```python
from build123d import *

# Parameters (mm, degrees)
BOSS_EXTRUDE1_DEPTH  = 25
CUT_EXTRUDE1_DEPTH   = 23
BOSS_EXTRUDE2_DEPTH  = 30
RIB5_REACH           = 157.804
SKETCH9_WALL_W       = 390.44961144
SKETCH9_WALL_H       = 50
FILLET2_R            = 2
FILLET3_R            = 2
FILLET2_OF_MIRROR1_R = 2
FILLET3_OF_MIRROR1_R = 2
RIB6_REACH           = 157.804
SKETCH10_WALL_W      = 362.214279798
SKETCH10_WALL_H      = 90
FILLET4_R            = 2
FILLET4_OF_MIRROR3_R = 2
SKETCH11_W           = 95
SKETCH11_H           = 63
CUT_EXTRUDE2_DEPTH   = 30
CUT_EXTRUDE3_DEPTH   = 1
SKETCH14_R           = 9
CUT_EXTRUDE4_DEPTH   = 5
FILLET6_R            = 3
FILLET7_R            = 3
CUT_EXTRUDE5_REACH   = 157.804
SKETCH21_R           = 3


with BuildPart() as part:
    # Sketch1 → Boss-Extrude1 (new body)
    with BuildSketch(Plane.XY):
        with BuildLine():
            Line((-119, 35), (-58.5, 35))
            ThreePointArc((-58.5, 35), (-54.257359313, 36.757359313), (-52.5, 41))
            Line((-52.5, 41), (-52.5, 69))
            ThreePointArc((-52.5, 69), (-50.742640687, 73.242640687), (-46.5, 75))
            Line((-46.5, 75), (46.5, 75))
            ThreePointArc((46.5, 75), (50.742640687, 73.242640687), (52.5, 69))
            Line((52.5, 69), (52.5, 41))
            ThreePointArc((52.5, 41), (54.257359313, 36.757359313), (58.5, 35))
            Line((58.5, 35), (119, 35))
            ThreePointArc((119, 35), (123.242640687, 33.242640687), (125, 29))
            Line((125, 29), (125, -29))
            ThreePointArc((125, -29), (123.242640687, -33.242640687), (119, -35))
            Line((119, -35), (58.5, -35))
            ThreePointArc((58.5, -35), (54.257359313, -36.757359313), (52.5, -41))
            Line((52.5, -41), (52.5, -69))
            ThreePointArc((52.5, -69), (50.742640687, -73.242640687), (46.5, -75))
            Line((46.5, -75), (-46.5, -75))
            ThreePointArc((-46.5, -75), (-50.742640687, -73.242640687), (-52.5, -69))
            Line((-52.5, -69), (-52.5, -41))
            ThreePointArc((-52.5, -41), (-54.257359313, -36.757359313), (-58.5, -35))
            Line((-58.5, -35), (-119, -35))
            ThreePointArc((-119, -35), (-123.242640687, -33.242640687), (-125, -29))
            Line((-125, -29), (-125, 29))
            ThreePointArc((-125, 29), (-123.242640687, 33.242640687), (-119, 35))
        make_face()
    extrude(amount=BOSS_EXTRUDE1_DEPTH)

    # Sketch2 → Cut-Extrude1 (cut)
    with BuildSketch(Plane(origin=(0, 0, 0), x_dir=(-1, 0, 0), z_dir=(0, 0, -1))):
        with BuildLine():
            Line((41.5, -65), (-41.5, -65))
            ThreePointArc((-41.5, -65), (-45.742640687, -63.242640687), (-47.5, -59))
            Line((-47.5, -59), (-47.5, -37.5))
            ThreePointArc((-47.5, -37.5), (-49.257359313, -33.257359313), (-53.5, -31.5))
            Line((-53.5, -31.5), (-108.997872355, -31.5))
            ThreePointArc((-108.997872355, -31.5), (-113.240513042, -29.742640687), (-114.997872355, -25.5))
            Line((-114.997872355, -25.5), (-114.997872355, 25.5))
            ThreePointArc((-114.997872355, 25.5), (-113.240513042, 29.742640687), (-108.997872355, 31.5))
            Line((-108.997872355, 31.5), (-53.5, 31.5))
            ThreePointArc((-53.5, 31.5), (-49.257359313, 33.257359313), (-47.5, 37.5))
            Line((-47.5, 37.5), (-47.5, 59))
            ThreePointArc((-47.5, 59), (-45.742640687, 63.242640687), (-41.5, 65))
            Line((-41.5, 65), (41.5, 65))
            ThreePointArc((41.5, 65), (45.742640687, 63.242640687), (47.5, 59))
            Line((47.5, 59), (47.5, 37.5))
            ThreePointArc((47.5, 37.5), (49.257359313, 33.257359313), (53.5, 31.5))
            Line((53.5, 31.5), (108.997872355, 31.5))
            ThreePointArc((108.997872355, 31.5), (113.240513042, 29.742640687), (114.997872355, 25.5))
            Line((114.997872355, 25.5), (114.997872355, -25.5))
            ThreePointArc((114.997872355, -25.5), (113.240513042, -29.742640687), (108.997872355, -31.5))
            Line((108.997872355, -31.5), (53.5, -31.5))
            ThreePointArc((53.5, -31.5), (49.257359313, -33.257359313), (47.5, -37.5))
            Line((47.5, -37.5), (47.5, -59))
            ThreePointArc((47.5, -59), (45.742640687, -63.242640687), (41.5, -65))
        make_face()
    extrude(amount=-CUT_EXTRUDE1_DEPTH, mode=Mode.SUBTRACT)

    # Sketch3 → Boss-Extrude2 (add)
    with BuildSketch(Plane.XY.offset(25)):
        with BuildLine():
            Line((-48.257359313, 36.757359313), (48.257359313, 36.757359313))
            ThreePointArc((48.257359313, 36.757359313), (52.5, 35), (54.257359313, 30.757359313))
            Line((54.257359313, 30.757359313), (54.257359313, -30.757359313))
            ThreePointArc((54.257359313, -30.757359313), (52.5, -35), (48.257359313, -36.757359313))
            Line((48.257359313, -36.757359313), (-48.257359313, -36.757359313))
            ThreePointArc((-48.257359313, -36.757359313), (-52.5, -35), (-54.257359313, -30.757359313))
            Line((-54.257359313, -30.757359313), (-54.257359313, 30.757359313))
            ThreePointArc((-54.257359313, 30.757359313), (-52.5, 35), (-48.257359313, 36.757359313))
        make_face()
    extrude(amount=BOSS_EXTRUDE2_DEPTH)

    # Sketch9 wall → Rib5 (add, up to next)
    with BuildSketch(Plane(origin=(-89.628679656, 0, 40), x_dir=(0.920638056948, 0, 0.390417171881), z_dir=(0.390417171881, 0, -0.920638056948)), mode=Mode.PRIVATE) as rib5_sk1:
        Rectangle(SKETCH9_WALL_W, SKETCH9_WALL_H)
    rib5_tool1 = extrude(rib5_sk1.sketch, amount=RIB5_REACH, mode=Mode.PRIVATE) - part.part
    rib5 = rib5_tool1.solids().sort_by_distance((-89.628679656, 0, 40))[0]
    add(rib5)

    # Fillet2
    fillet2_edges = [part.edges().sort_by_distance(p)[0] for p in [
        (-89.628679656, -25, 40),
    ]]
    fillet(fillet2_edges, radius=FILLET2_R)

    # Fillet3
    fillet3_edges = [part.edges().sort_by_distance(p)[0] for p in [
        (-89.628679656, 25, 40),
    ]]
    fillet(fillet3_edges, radius=FILLET3_R)

    # Mirror1: Rib5 across plane
    add(rib5.mirror(Plane(origin=(0, 0, 0), x_dir=(0, 0, 1), z_dir=(1, 0, 0))))

    # Fillet2 of Mirror1
    fillet2_of_mirror1_edges = [part.edges().sort_by_distance(p)[0] for p in [
        (89.628679656, -25, 40),
    ]]
    fillet(fillet2_of_mirror1_edges, radius=FILLET2_OF_MIRROR1_R)

    # Fillet3 of Mirror1
    fillet3_of_mirror1_edges = [part.edges().sort_by_distance(p)[0] for p in [
        (89.628679656, 25, 40),
    ]]
    fillet(fillet3_of_mirror1_edges, radius=FILLET3_OF_MIRROR1_R)

    # Sketch10 wall → Rib6 (add, up to next)
    with BuildSketch(Plane(origin=(0, 55.878679656, 40), x_dir=(0, 0.78679574807, -0.617213456447), z_dir=(0, 0.617213456447, 0.78679574807)), mode=Mode.PRIVATE) as rib6_sk1:
        Rectangle(SKETCH10_WALL_W, SKETCH10_WALL_H)
    rib6_tool1 = extrude(rib6_sk1.sketch, amount=-RIB6_REACH, mode=Mode.PRIVATE) - part.part
    rib6 = rib6_tool1.solids().sort_by_distance((0, 55.878679656, 40))[0]
    add(rib6)

    # Fillet4
    fillet4_edges = [part.edges().sort_by_distance(p)[0] for p in [
        (45, 55.878679656, 40),
        (-45, 55.878679656, 40),
    ]]
    fillet(fillet4_edges, radius=FILLET4_R)

    # Mirror3: Rib6 across plane
    add(rib6.mirror(Plane.ZX))

    # Fillet4 of Mirror3
    fillet4_of_mirror3_edges = [part.edges().sort_by_distance(p)[0] for p in [
        (45, -55.878679656, 40),
        (-45, -55.878679656, 40),
    ]]
    fillet(fillet4_of_mirror3_edges, radius=FILLET4_OF_MIRROR3_R)

    # Sketch11 → Cut-Extrude2 (cut)
    with BuildSketch(Plane(origin=(0, 0, 23), x_dir=(-1, 0, 0), z_dir=(0, 0, -1))):
        Rectangle(SKETCH11_W, SKETCH11_H)
    extrude(amount=-CUT_EXTRUDE2_DEPTH, mode=Mode.SUBTRACT)

    # Sketch12 → Cut-Extrude3 (cut)
    with BuildSketch(Plane.XY.offset(55)):
        with BuildLine():
            Line((6, 25), (6, -25))
            ThreePointArc((6, -25), (0, -31), (-6, -25))
            Line((-6, -25), (-6, 25))
            ThreePointArc((-6, 25), (0, 31), (6, 25))
        make_face()
        with BuildLine():
            Line((21, 25), (21, -25))
            ThreePointArc((21, -25), (15, -31), (9, -25))
            Line((9, -25), (9, 25))
            ThreePointArc((9, 25), (15, 31), (21, 25))
        make_face()
        with BuildLine():
            Line((36, 25), (36, -25))
            ThreePointArc((36, -25), (30, -31), (24, -25))
            Line((24, -25), (24, 25))
            ThreePointArc((24, 25), (30, 31), (36, 25))
        make_face()
        with BuildLine():
            Line((51, 25), (51, -25))
            ThreePointArc((51, -25), (45, -31), (39, -25))
            Line((39, -25), (39, 25))
            ThreePointArc((39, 25), (45, 31), (51, 25))
        make_face()
        with BuildLine():
            Line((-51, 25), (-51, -25))
            ThreePointArc((-51, -25), (-45, -31), (-39, -25))
            Line((-39, -25), (-39, 25))
            ThreePointArc((-39, 25), (-45, 31), (-51, 25))
        make_face()
        with BuildLine():
            Line((-36, 25), (-36, -25))
            ThreePointArc((-36, -25), (-30, -31), (-24, -25))
            Line((-24, -25), (-24, 25))
            ThreePointArc((-24, 25), (-30, 31), (-36, 25))
        make_face()
        with BuildLine():
            Line((-21, 25), (-21, -25))
            ThreePointArc((-21, -25), (-15, -31), (-9, -25))
            Line((-9, -25), (-9, 25))
            ThreePointArc((-9, 25), (-15, 31), (-21, 25))
        make_face()
    extrude(amount=-CUT_EXTRUDE3_DEPTH, mode=Mode.SUBTRACT)

    # Sketch14 → Cut-Extrude4 (cut)
    with BuildSketch(Plane.ZY.offset(125)):
        with Locations((12.5, 14)):
            Circle(SKETCH14_R)
        with Locations((12.5, -14)):
            Circle(SKETCH14_R)
    extrude(amount=-CUT_EXTRUDE4_DEPTH, mode=Mode.SUBTRACT)

    # Fillet6
    fillet6_edges = [part.edges().sort_by_distance(p)[0] for p in [
        (-120, 14, 3.5),
    ]]
    fillet(fillet6_edges, radius=FILLET6_R)

    # Fillet7
    fillet7_edges = [part.edges().sort_by_distance(p)[0] for p in [
        (-120, -14, 3.5),
    ]]
    fillet(fillet7_edges, radius=FILLET7_R)

    # Sketch21 → Cut-Extrude5 (cut, up to next)
    with BuildSketch(Plane.XY.offset(55), mode=Mode.PRIVATE) as cut_extrude5_sk1:
        with Locations((-38, 70)):
            Circle(SKETCH21_R)
    cut_extrude5_tool1 = extrude(cut_extrude5_sk1.sketch, amount=-CUT_EXTRUDE5_REACH, mode=Mode.PRIVATE) & part.part
    # Sketch21 → Cut-Extrude5 (cut, up to next)
    with BuildSketch(Plane.XY.offset(55), mode=Mode.PRIVATE) as cut_extrude5_sk2:
        with Locations((38, 70)):
            Circle(SKETCH21_R)
    cut_extrude5_tool2 = extrude(cut_extrude5_sk2.sketch, amount=-CUT_EXTRUDE5_REACH, mode=Mode.PRIVATE) & part.part
    # Sketch21 → Cut-Extrude5 (cut, up to next)
    with BuildSketch(Plane.XY.offset(55), mode=Mode.PRIVATE) as cut_extrude5_sk3:
        with Locations((38, -70)):
            Circle(SKETCH21_R)
    cut_extrude5_tool3 = extrude(cut_extrude5_sk3.sketch, amount=-CUT_EXTRUDE5_REACH, mode=Mode.PRIVATE) & part.part
    # Sketch21 → Cut-Extrude5 (cut, up to next)
    with BuildSketch(Plane.XY.offset(55), mode=Mode.PRIVATE) as cut_extrude5_sk4:
        with Locations((-38, -70)):
            Circle(SKETCH21_R)
    cut_extrude5_tool4 = extrude(cut_extrude5_sk4.sketch, amount=-CUT_EXTRUDE5_REACH, mode=Mode.PRIVATE) & part.part
    # Sketch21 → Cut-Extrude5 (cut, up to next)
    with BuildSketch(Plane.XY.offset(55), mode=Mode.PRIVATE) as cut_extrude5_sk5:
        with Locations((-120, 0)):
            Circle(SKETCH21_R)
    cut_extrude5_tool5 = extrude(cut_extrude5_sk5.sketch, amount=-CUT_EXTRUDE5_REACH, mode=Mode.PRIVATE) & part.part
    # Sketch21 → Cut-Extrude5 (cut, up to next)
    with BuildSketch(Plane.XY.offset(55), mode=Mode.PRIVATE) as cut_extrude5_sk6:
        with Locations((120, 0)):
            Circle(SKETCH21_R)
    cut_extrude5_tool6 = extrude(cut_extrude5_sk6.sketch, amount=-CUT_EXTRUDE5_REACH, mode=Mode.PRIVATE) & part.part
    add(cut_extrude5_tool1.solids().sort_by_distance((-38, 70, 55))[0], mode=Mode.SUBTRACT)
    add(cut_extrude5_tool2.solids().sort_by_distance((38, 70, 55))[0], mode=Mode.SUBTRACT)
    add(cut_extrude5_tool3.solids().sort_by_distance((38, -70, 55))[0], mode=Mode.SUBTRACT)
    add(cut_extrude5_tool4.solids().sort_by_distance((-38, -70, 55))[0], mode=Mode.SUBTRACT)
    add(cut_extrude5_tool5.solids().sort_by_distance((-120, 0, 55))[0], mode=Mode.SUBTRACT)
    add(cut_extrude5_tool6.solids().sort_by_distance((120, 0, 55))[0], mode=Mode.SUBTRACT)


solid = part.part
```
Design review of the part built by this model. Coordinates are the model's own, in mm. A direction names the side the tool comes from. Round coordinates to 2 decimals unless told otherwise and drop trailing zeros. Write each loop counter-clockwise with the first axis right and the second up, starting at its lowest first coordinate (ties: lowest second). Pieces come first, ordered by that corner, then holes. Notation, with made-up numbers: (62.5, -5.5) -> (81.5, -5.5) arc R25 ccw to (81.5, 14.5) -> close; hole circle Ø7 at (13.5, 50). An arc over 180 degrees is marked (long way). Answer in a Markdown table with one row per item.
Q1. For faces 1 (the face through (-76, -25, 33)), 2 (the face through (-124.01, 8.52, 5.36)), 3 (the face through (-49.304, -33.211, 11.339)), 4 (the face through (54.257, 28, 40)), list the 3-axis set-ups (+Z, -Z, +X, -X, +Y, -Y) from which the entire face can be reached by the end or side of a thin tool; tool diameter is ignored.
The answers:
| item | result |
|---|---|
| face 1 | +Z, -X, -Y |
| face 2 | -X |
| face 3 | -Z |
| face 4 | +Z, +X, +Y |
Q2. To check wall thickness, follow L1, parallel to Y at x = 38, z = 12; L2, parallel to X at y = 0, z = 10; L3, parallel to X at y = 4.5, z = 13.5. State the ranges of each line that lie inside material, in increasing order. Write a range as [from, to].
The answers:
| item | result |
|---|---|
| L1 | [-75, -73], [-67, -65], [65, 67], [73, 75] |
| L2 | [-125, -123], [-117, -115], [115, 117], [123, 125] |
| L3 | [-125, -115], [115, 125] |
Q3. Draft analysis for pull direction X (two halves, no side actions). For faces 5 (the face through (-49.211, 33.304, 11.339)), 6 (the face through (78, -33, 25)), 7 (the face through (-52.5, 35, 39.8)), state which applies: +X half, -X half, draft (parallel to the pull), parting line (faces both ways), or undercut.
The answers:
| item | result |
|---|---|
| face 5 | undercut |
| face 6 | draft |
| face 7 | -X half |
Q4. Take a section at A-A, the plane x = 15. State the section outline as (y, z) points, then the cut area to 3 significant figures.
The answers:
| item | result |
|---|---|
| outline | (-75, 0) -> (-65, 0) -> (-65, 23) -> (-31.5, 23) -> (-31.5, 53) -> (31.5, 53) -> (31.5, 23) -> (65, 23) -> (65, 0) -> (75, 0) -> (75, 25) -> (36.76, 55) -> (31, 55) -> (31, 54) -> (-31, 54) -> (-31, 55) -> (-36.76, 55) -> (-75, 25) -> close |
| area | 2,160 mm² |
Q5. Clearance check with flat-ended pins moving along their axes: pin 1 Ø6 at (x, z) = (-88.5, 34) entering from -Y; pin 2 Ø11 at (y, z) = (-45, 9) entering from +X; pin 3 Ø4 at (x, z) = (75, 45.5) entering from +Y; pin 4 Ø5.5 at (x, y) = (-38, -70) entering from -Z. State where each tip first meets the part, or that it passes through.
The answers:
| item | result |
|---|---|
| pin 1 | y = -25 |
| pin 2 | x = 52.69 |
| pin 3 | y = 25 |
| pin 4 | through |
Q6. Take a section at B-B, the plane z = 12.5. Count the separate pieces of the cut face and the enclosed holes in it, then the cut area to 3 significant figures.
The answers:
| item | result |
|---|---|
| separate pieces | 1 |
| enclosed holes | 7 |
| area | 4,700 mm² |
